CAD build for the part. Positions are in the model's coordinates, mm. Face numbers are marked on the shaded views. A direction names the side the tool comes from. Give positions to 0.01 mm unless a question says otherwise; leave off trailing zeros. Loops run counter-clockwise (first coordinate to the right, second up) from the corner with the lowest first, then second, coordinate; pieces in that order, holes last.
Item 1: Saw through at A-A on z = -9. Give the cut face in (x, y), plus the area to 3 significant figures.
Item 2: Saw through at C-C on x = 2. Give the cut face in (y, z), plus the area to 3 significant figures.
Item 3: Saw through at D-D on y = 7.5. Give the cut face in (x, z), plus the area to 3 significant figures.
Item 4: Which spindle directions (+Z, -Z, +X, -X, +Y, -Y) get a long thin tool onto all of the face, cutting with end or side? Do the marked faces 1, 2, 3, 4 and 5. Say none if no direction does.
Item 5: Probe probe 1 along Y at (x, z) = (1.75, -28.5); probe 2 along Z at (x, y) = (12.5, 13). List the from-to ranges inside material, lowest first.
Item 6: Saw through at B-B on z = -3.5. Give the cut face in (x, y), plus the area to 3 significant figures.
Item 7: Mould opens along X. For the marked faces 6, 7 and 8 say: released by +X, released by -X, zero draft, split by the parting line, or undercut.
Item 8: Drop flat-ended pins along their axis: P1, Ø6, axis at y = 24.5, z = -7.5, coming from the +X side; P2, Ø5, axis at x = 7, z = -15, coming from the +Y side; P3, Ø3, axis at x = 18.5, y = 24.5, coming from the +Z side. Give the stop position or say it passes through.
from build123d import *

# Parameters (mm, degrees)
SKETCH_1_W           = 30
SKETCH_1_H           = 30
EXTRUDE_1_DEPTH      = 30
SKETCH_30_W          = 10
SKETCH_30_H          = 10
SKETCH_30_H_2        = 20
CUT_EXTRUDE_20_DEPTH = 52.961524227
SKETCH_32_W          = 10
SKETCH_32_H          = 10
CUT_EXTRUDE_21_DEPTH = 47.904157598
SKETCH_33_W          = 10
SKETCH_33_H          = 10
CUT_EXTRUDE_22_DEPTH = 52.961524227


with BuildPart() as part:
    # 草圖1 → 填料-伸1 (new body)
    with BuildSketch(Plane.XY):
        with Locations((15, 15)):
            Rectangle(SKETCH_1_W, SKETCH_1_H)
    extrude(amount=-EXTRUDE_1_DEPTH)

    # 草圖30 → 除料-伸長20 (cut, through all)
    with BuildSketch(Plane.XY):
        with Locations((5, 25)):
            Rectangle(SKETCH_30_W, SKETCH_30_H)
        with Locations((25, 20)):
            Rectangle(SKETCH_30_W, SKETCH_30_H_2)
    extrude(amount=-CUT_EXTRUDE_20_DEPTH, mode=Mode.SUBTRACT)

    # 草圖32 → 除料-伸長21 (cut, through all)
    with BuildSketch(Plane(origin=(20, 0, 0), x_dir=(0, 0, -1), z_dir=(1, 0, 0))):
        with Locations((5, 25)):
            Rectangle(SKETCH_32_W, SKETCH_32_H)
        Polygon((0, 10), (10, 20), (0, 20), align=None)
    extrude(amount=-CUT_EXTRUDE_21_DEPTH, mode=Mode.SUBTRACT)

    # 草圖33 → 除料-伸長22 (cut, through all)
    with BuildSketch(Plane(origin=(0, 30, 0), x_dir=(1, 0, 0), z_dir=(0, 1, 0))):
        with Locations((15, 5)):
            Rectangle(SKETCH_33_W, SKETCH_33_H)
        Polygon((30, 10), (20, 0), (30, 0), align=None)
    extrude(amount=-CUT_EXTRUDE_22_DEPTH, mode=Mode.SUBTRACT)


solid = part.part
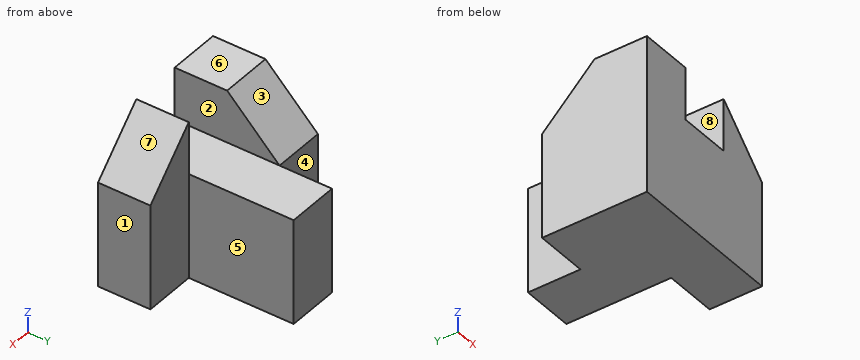
Results below:
1. outline: (0, 0) - (10, 0) - (10, 19) - (0, 19) - close; (20, 0) - (29, 0) - (29, 10) - (20, 10) - close
1. area: 280 mm2
2. outline: (0, -30) - (20, -30) - (20, -10) - (10, 0) - (0, 0) - close
2. area: 550 mm2
3. outline: (0, -30) - (30, -30) - (30, -10) - (20, 0) - (20, -10) - (10, -10) - (10, 0) - (0, 0) - close
3. area: 750 mm2
4. face 1: +Z, -Z, +X, +Y, -Y
4. face 2: +Z, +Y, -Y
4. face 3: +Z, +X, -X, +Y
4. face 4: +Z, -Z, -X, +Y
4. face 5: +Z, -Z, +X, +Y
5. probe 1: y = 0 to 20
5. probe 2: z = -30 to -10
6. outline: (0, 0) - (10, 0) - (10, 13.5) - (0, 13.5) - close; (20, 0) - (23.5, 0) - (23.5, 10) - (20, 10) - close
6. area: 170 mm2
7. face 6: zero draft
7. face 7: released by +X
7. face 8: undercut
8. P1: stops at x = 20
8. P2: stops at y = 20
8. P3: stops at z = -10
